Geometry: final body of the model. Coordinates: model frame, mm. A direction names the side the tool comes from. Coordinates: 2 decimals unless noted, no trailing zeros. Write item = value, one per line.
from build123d import *

# Parameters (mm, degrees)
SKETCH1_R           = 1.65
BOSS_EXTRUDE1_DEPTH = 6
CHAMFER1_SIZE       = 1.1
FILLET1_R           = 1


with BuildPart() as part:
    # Sketch1 → Boss-Extrude1 (new body)
    with BuildSketch(Plane.XY):
        with BuildLine():
            Line((1, 6), (1, 346))
            ThreePointArc((1, 346), (2.464466094, 349.535533906), (6, 351))
            Line((6, 351), (186, 351))
            ThreePointArc((186, 351), (189.535533906, 349.535533906), (191, 346))
            Line((191, 346), (191, 6))
            ThreePointArc((191, 6), (189.535533906, 2.464466094), (186, 1))
            Line((186, 1), (6, 1))
            ThreePointArc((6, 1), (2.464466094, 2.464466094), (1, 6))
        make_face()
        with Locations((7, 345)):
            Circle(SKETCH1_R, mode=Mode.SUBTRACT)
        with Locations((185, 345)):
            Circle(SKETCH1_R, mode=Mode.SUBTRACT)
        with Locations((7, 7)):
            Circle(SKETCH1_R, mode=Mode.SUBTRACT)
        with Locations((185, 7)):
            Circle(SKETCH1_R, mode=Mode.SUBTRACT)
        with Locations((7, 176)):
            Circle(SKETCH1_R, mode=Mode.SUBTRACT)
        with Locations((185, 176)):
            Circle(SKETCH1_R, mode=Mode.SUBTRACT)
        with BuildLine():
            Line((123.902123688, 337), (123.902123688, 184))
            ThreePointArc((123.902123688, 184), (125.902123688, 182), (127.902123688, 184))
            Line((127.902123688, 184), (127.902123688, 337))
            ThreePointArc((127.902123688, 337), (125.902123688, 339), (123.902123688, 337))
        make_face(mode=Mode.SUBTRACT)
        with BuildLine():
            ThreePointArc((55.902123688, 337), (53.902123688, 339), (51.902123688, 337))
            Line((51.902123688, 337), (51.902123688, 184))
            ThreePointArc((51.902123688, 184), (53.902123688, 182), (55.902123688, 184))
            Line((55.902123688, 184), (55.902123688, 337))
        make_face(mode=Mode.SUBTRACT)
        with BuildLine():
            Line((175.902123688, 337), (175.902123688, 184))
            ThreePointArc((175.902123688, 184), (173.902123688, 182), (171.902123688, 184))
            Line((171.902123688, 184), (171.902123688, 337))
            ThreePointArc((171.902123688, 337), (173.902123688, 339), (175.902123688, 337))
        make_face(mode=Mode.SUBTRACT)
        with BuildLine():
            Line((163.902123688, 337), (163.902123688, 184))
            ThreePointArc((163.902123688, 184), (161.902123688, 182), (159.902123688, 184))
            Line((159.902123688, 184), (159.902123688, 337))
            ThreePointArc((159.902123688, 337), (161.902123688, 339), (163.902123688, 337))
        make_face(mode=Mode.SUBTRACT)
        with BuildLine():
            Line((151.902123688, 337), (151.902123688, 184))
            ThreePointArc((151.902123688, 184), (149.902123688, 182), (147.902123688, 184))
            Line((147.902123688, 184), (147.902123688, 337))
            ThreePointArc((147.902123688, 337), (149.902123688, 339), (151.902123688, 337))
        make_face(mode=Mode.SUBTRACT)
        with BuildLine():
            Line((139.902123688, 337), (139.902123688, 184))
            ThreePointArc((139.902123688, 184), (137.902123688, 182), (135.902123688, 184))
            Line((135.902123688, 184), (135.902123688, 337))
            ThreePointArc((135.902123688, 337), (137.902123688, 339), (139.902123688, 337))
        make_face(mode=Mode.SUBTRACT)
        with BuildLine():
            Line((115.902123688, 337), (115.902123688, 184))
            ThreePointArc((115.902123688, 184), (113.902123688, 182), (111.902123688, 184))
            Line((111.902123688, 184), (111.902123688, 337))
            ThreePointArc((111.902123688, 337), (113.902123688, 339), (115.902123688, 337))
        make_face(mode=Mode.SUBTRACT)
        with BuildLine():
            Line((99.902123688, 337), (99.902123688, 184))
            ThreePointArc((99.902123688, 184), (101.902123688, 182), (103.902123688, 184))
            Line((103.902123688, 184), (103.902123688, 337))
            ThreePointArc((103.902123688, 337), (101.902123688, 339), (99.902123688, 337))
        make_face(mode=Mode.SUBTRACT)
        with BuildLine():
            Line((91.902123688, 337), (91.902123688, 184))
            ThreePointArc((91.902123688, 184), (89.902123688, 182), (87.902123688, 184))
            Line((87.902123688, 184), (87.902123688, 337))
            ThreePointArc((87.902123688, 337), (89.902123688, 339), (91.902123688, 337))
        make_face(mode=Mode.SUBTRACT)
        with BuildLine():
            Line((79.902123688, 337), (79.902123688, 184))
            ThreePointArc((79.902123688, 184), (77.902123688, 182), (75.902123688, 184))
            Line((75.902123688, 184), (75.902123688, 337))
            ThreePointArc((75.902123688, 337), (77.902123688, 339), (79.902123688, 337))
        make_face(mode=Mode.SUBTRACT)
        with BuildLine():
            Line((63.902123688, 337), (63.902123688, 184))
            ThreePointArc((63.902123688, 184), (65.902123688, 182), (67.902123688, 184))
            Line((67.902123688, 184), (67.902123688, 337))
            ThreePointArc((67.902123688, 337), (65.902123688, 339), (63.902123688, 337))
        make_face(mode=Mode.SUBTRACT)
        with BuildLine():
            Line((43.902123688, 337), (43.902123688, 184))
            ThreePointArc((43.902123688, 184), (41.902123688, 182), (39.902123688, 184))
            Line((39.902123688, 184), (39.902123688, 337))
            ThreePointArc((39.902123688, 337), (41.902123688, 339), (43.902123688, 337))
        make_face(mode=Mode.SUBTRACT)
        with BuildLine():
            Line((19.902123688, 337), (19.902123688, 184))
            ThreePointArc((19.902123688, 184), (17.902123688, 182), (15.902123688, 184))
            Line((15.902123688, 184), (15.902123688, 337))
            ThreePointArc((15.902123688, 337), (17.902123688, 339), (19.902123688, 337))
        make_face(mode=Mode.SUBTRACT)
        with BuildLine():
            Line((27.902123688, 337), (27.902123688, 184))
            ThreePointArc((27.902123688, 184), (29.902123688, 182), (31.902123688, 184))
            Line((31.902123688, 184), (31.902123688, 337))
            ThreePointArc((31.902123688, 337), (29.902123688, 339), (27.902123688, 337))
        make_face(mode=Mode.SUBTRACT)
        with BuildLine():
            Line((171.902123688, 15), (171.902123688, 168))
            ThreePointArc((171.902123688, 168), (173.902123688, 170), (175.902123688, 168))
            Line((175.902123688, 168), (175.902123688, 15))
            ThreePointArc((175.902123688, 15), (173.902123688, 13), (171.902123688, 15))
        make_face(mode=Mode.SUBTRACT)
        with BuildLine():
            Line((159.902123688, 15), (159.902123688, 168))
            ThreePointArc((159.902123688, 168), (161.902123688, 170), (163.902123688, 168))
            Line((163.902123688, 168), (163.902123688, 15))
            ThreePointArc((163.902123688, 15), (161.902123688, 13), (159.902123688, 15))
        make_face(mode=Mode.SUBTRACT)
        with BuildLine():
            Line((147.902123688, 15), (147.902123688, 168))
            ThreePointArc((147.902123688, 168), (149.902123688, 170), (151.902123688, 168))
            Line((151.902123688, 168), (151.902123688, 15))
            ThreePointArc((151.902123688, 15), (149.902123688, 13), (147.902123688, 15))
        make_face(mode=Mode.SUBTRACT)
        with BuildLine():
            Line((135.902123688, 15), (135.902123688, 168))
            ThreePointArc((135.902123688, 168), (137.902123688, 170), (139.902123688, 168))
            Line((139.902123688, 168), (139.902123688, 15))
            ThreePointArc((139.902123688, 15), (137.902123688, 13), (135.902123688, 15))
        make_face(mode=Mode.SUBTRACT)
        with BuildLine():
            Line((123.902123688, 15), (123.902123688, 168))
            ThreePointArc((123.902123688, 168), (125.902123688, 170), (127.902123688, 168))
            Line((127.902123688, 168), (127.902123688, 15))
            ThreePointArc((127.902123688, 15), (125.902123688, 13), (123.902123688, 15))
        make_face(mode=Mode.SUBTRACT)
        with BuildLine():
            Line((111.902123688, 15), (111.902123688, 168))
            ThreePointArc((111.902123688, 168), (113.902123688, 170), (115.902123688, 168))
            Line((115.902123688, 168), (115.902123688, 15))
            ThreePointArc((115.902123688, 15), (113.902123688, 13), (111.902123688, 15))
        make_face(mode=Mode.SUBTRACT)
        with BuildLine():
            Line((99.902123688, 15), (99.902123688, 168))
            ThreePointArc((99.902123688, 168), (101.902123688, 170), (103.902123688, 168))
            Line((103.902123688, 168), (103.902123688, 15))
            ThreePointArc((103.902123688, 15), (101.902123688, 13), (99.902123688, 15))
        make_face(mode=Mode.SUBTRACT)
        with BuildLine():
            Line((87.902123688, 15), (87.902123688, 168))
            ThreePointArc((87.902123688, 168), (89.902123688, 170), (91.902123688, 168))
            Line((91.902123688, 168), (91.902123688, 15))
            ThreePointArc((91.902123688, 15), (89.902123688, 13), (87.902123688, 15))
        make_face(mode=Mode.SUBTRACT)
        with BuildLine():
            Line((75.902123688, 15), (75.902123688, 168))
            ThreePointArc((75.902123688, 168), (77.902123688, 170), (79.902123688, 168))
            Line((79.902123688, 168), (79.902123688, 15))
            ThreePointArc((79.902123688, 15), (77.902123688, 13), (75.902123688, 15))
        make_face(mode=Mode.SUBTRACT)
        with BuildLine():
            Line((63.902123688, 15), (63.902123688, 168))
            ThreePointArc((63.902123688, 168), (65.902123688, 170), (67.902123688, 168))
            Line((67.902123688, 168), (67.902123688, 15))
            ThreePointArc((67.902123688, 15), (65.902123688, 13), (63.902123688, 15))
        make_face(mode=Mode.SUBTRACT)
        with BuildLine():
            Line((51.902123688, 15), (51.902123688, 168))
            ThreePointArc((51.902123688, 168), (53.902123688, 170), (55.902123688, 168))
            Line((55.902123688, 168), (55.902123688, 15))
            ThreePointArc((55.902123688, 15), (53.902123688, 13), (51.902123688, 15))
        make_face(mode=Mode.SUBTRACT)
        with BuildLine():
            Line((39.902123688, 15), (39.902123688, 168))
            ThreePointArc((39.902123688, 168), (41.902123688, 170), (43.902123688, 168))
            Line((43.902123688, 168), (43.902123688, 15))
            ThreePointArc((43.902123688, 15), (41.902123688, 13), (39.902123688, 15))
        make_face(mode=Mode.SUBTRACT)
        with BuildLine():
            Line((27.902123688, 15), (27.902123688, 168))
            ThreePointArc((27.902123688, 168), (29.902123688, 170), (31.902123688, 168))
            Line((31.902123688, 168), (31.902123688, 15))
            ThreePointArc((31.902123688, 15), (29.902123688, 13), (27.902123688, 15))
        make_face(mode=Mode.SUBTRACT)
        with BuildLine():
            Line((19.902123688, 15), (19.902123688, 168))
            ThreePointArc((19.902123688, 168), (17.902123688, 170), (15.902123688, 168))
            Line((15.902123688, 168), (15.902123688, 15))
            ThreePointArc((15.902123688, 15), (17.902123688, 13), (19.902123688, 15))
        make_face(mode=Mode.SUBTRACT)
    extrude(amount=BOSS_EXTRUDE1_DEPTH)

    # Chamfer1
    chamfer1_edges = [part.edges().sort_by_distance(p)[0] for p in [
        (5.35, 345, 0),
        (183.35, 345, 0),
        (5.35, 7, 0),
        (183.35, 7, 0),
        (5.35, 176, 0),
        (183.35, 176, 0),
    ]]
    chamfer(chamfer1_edges, length=CHAMFER1_SIZE)

    # Fillet1
    fillet1_edges = [part.edges().sort_by_distance(p)[0] for p in [
        (189.535533906, 349.535533906, 6),
        (96, 351, 6),
        (2.464466094, 349.535533906, 6),
        (1, 176, 6),
        (2.464466094, 2.464466094, 6),
        (96, 1, 6),
        (189.535533906, 2.464466094, 6),
        (191, 176, 6),
    ]]
    fillet(fillet1_edges, radius=FILLET1_R)


solid = part.part
1) Section A-A, the plane y = 221. Give the number of separate pieces and of enclosed holes in the cut face, and give its area (3 significant figures).
Numbers:
separate_pieces = 15
enclosed_holes = 0
area = 804 mm²
2) Mould query, pull axis Y, two halves, no side actions, for faces 3 (the face through (97, 178, 6)), 4 (the face through (67.902, 259, 3)), 5 (the face through (175.902, 93, 3)). Classes: pulls with the +Y half, pulls with the -Y half, needs draft (parallel to the pull), parting line crosses it, or undercut.
Numbers:
face_3 = needs draft
face_4 = undercut
face_5 = undercut
3) Line query: L1, parallel to X at y = 176, z = 3.95; L2, parallel to Y at x = 102, z = 3.25; L3, parallel to Y at x = 7, z = 2.9. Output: solid intervals per line, ascending.
Numbers:
L1 = 1 to 5.35, 8.65 to 183.35, 186.65 to 191
L2 = 1 to 13, 170 to 182, 339 to 351
L3 = 1 to 5.35, 8.65 to 174.35, 177.65 to 343.35, 346.65 to 351
4) Set-up query: faces 1 (the face through (97, 178, 0)), 2 (the face through (151.902, 93, 3)). Return all of +Z, -Z, +X, -X, +Y, -Y with unobstructed straight access to the full face (end or side cutting, diameter ignored); none if empty.
Numbers:
face_1 = -Z, +X, -X, +Y, -Y
face_2 = +Z, -Z
5) Pin query (flat end, axial travel): pin 1 (4 mm diameter, centred on x = 7, y = 176, fed in from -Z). Return the tip coordinate at first contact, or that it passes through.
Numbers:
pin_1 = 0.75
